from build123d import *

# Parameters (mm, degrees)
SKETCH1_W           = 80
SKETCH1_H           = 80
BOSS_EXTRUDE1_DEPTH = 2.5
SKETCH2_W           = 80
SKETCH2_H           = 80
SKETCH2_W_2         = 75
SKETCH2_H_2         = 75
BOSS_EXTRUDE2_DEPTH = 16
BOSS_EXTRUDE3_REACH = 93.336
SKETCH4_W           = 5
SKETCH4_H           = 2
CUT_EXTRUDE2_DEPTH  = 2.5


with BuildPart() as part:
    # Sketch1 → Boss-Extrude1 (new body)
    with BuildSketch(Plane(origin=(0, 0, 0), x_dir=(1, 0, 0), z_dir=(0, 1, 0))):
        Rectangle(SKETCH1_W, SKETCH1_H)
    extrude(amount=BOSS_EXTRUDE1_DEPTH)

    # Sketch2 → Boss-Extrude2 (add)
    with BuildSketch(Plane(origin=(0, 2.5, 0), x_dir=(1, 0, 0), z_dir=(0, 1, 0))):
        Rectangle(SKETCH2_W, SKETCH2_H)
        Rectangle(SKETCH2_W_2, SKETCH2_H_2, mode=Mode.SUBTRACT)
    extrude(amount=BOSS_EXTRUDE2_DEPTH)

    # Sketch4 → Boss-Extrude3 (add, up to next)
    with BuildSketch(Plane.XY.offset(40), mode=Mode.PRIVATE) as boss_extrude3_sk1:
        with Locations((-37.5, 17.5)):
            Rectangle(SKETCH4_W, SKETCH4_H)
    boss_extrude3_tool1 = extrude(boss_extrude3_sk1.sketch, amount=-BOSS_EXTRUDE3_REACH, mode=Mode.PRIVATE) - part.part
    # Sketch4 → Boss-Extrude3 (add, up to next)
    with BuildSketch(Plane.XY.offset(40), mode=Mode.PRIVATE) as boss_extrude3_sk2:
        with Locations((37.5, 17.5)):
            Rectangle(SKETCH4_W, SKETCH4_H)
    boss_extrude3_tool2 = extrude(boss_extrude3_sk2.sketch, amount=-BOSS_EXTRUDE3_REACH, mode=Mode.PRIVATE) - part.part
    add(boss_extrude3_tool1.solids().sort_by_distance((-37.5, 17.5, 40))[0])
    add(boss_extrude3_tool2.solids().sort_by_distance((37.5, 17.5, 40))[0])

    # Sketch5 → Cut-Extrude2 (cut)
    with BuildSketch(Plane(origin=(0, 0, -40), x_dir=(-1, 0, 0), z_dir=(0, 0, -1))):
        Polygon((-32.2, 18.5), (-35, 18.5), (-35, 16.5), (-37.5, 16.5), (-37.5, 14.2), (-32.2, 14.2), align=None)
        Polygon((35, 18.5), (32.2, 18.5), (32.2, 14.2), (37.5, 14.2), (37.5, 16.5), (35, 16.5), align=None)
    extrude(amount=-CUT_EXTRUDE2_DEPTH, mode=Mode.SUBTRACT)


solid = part.part
Could you check a few things on this model? Use its own coordinates, in mm. A direction names the side the tool comes from. Round coordinates to 2 decimals unless told otherwise and drop trailing zeros. Write each loop counter-clockwise with the first axis right and the second up, starting at its lowest first coordinate (ties: lowest second). Pieces come first, ordered by that corner, then holes. Notation, with made-up numbers: (0, 24.5) - (24, 24.5) arc R32 cw to (24, 59.5) - close; hole circle Ø9 at (-24, -33.75). An arc over 180 degrees is marked (long way). Use a Markdown table: item, result.
Q1. I want a section at B-B (x = 20.5). List the corners of the cut face in (y, z) for me, plus the area to 3 significant figures.
Output values:
| item | result |
|---|---|
| outline | (0, -40) - (18.5, -40) - (18.5, -37.5) - (2.5, -37.5) - (2.5, 37.5) - (18.5, 37.5) - (18.5, 40) - (0, 40) - close |
| area | 280 mm2 |
Q2. Thinking about a two-plate mould opening in Z: for faces 1 (the flat face through (-1, 9, 40)), 2 (the flat face through (40, 9, 1)), 3 (the flat face through (-37.5, 9, -1)), which applies, released by +Z, released by -Z, zero draft, split by the parting line, or undercut?
Output values:
| item | result |
|---|---|
| face 1 | released by +Z |
| face 2 | zero draft |
| face 3 | undercut |
Q3. I want a section at A-A (y = 11.75). List the corners of the cut face in (x, z) for me.
Output values:
| item | result |
|---|---|
| outline | (-40, -40) - (40, -40) - (40, 40) - (-40, 40) - close; hole (-37.5, -37.5) - (37.5, -37.5) - (37.5, 37.5) - (-37.5, 37.5) - close |
Q4. For faces 4 (the flat face through (-35, 14.2, -39)), 5 (the flat face through (-40, 9, 1)), 6 (the flat face through (32.2, 16, -39)), which set-ups out of +Z, -Z, +X, -X, +Y, -Y let a thin tool reach every point of the face, with its end or its side?
Output values:
| item | result |
|---|---|
| face 4 | -Z |
| face 5 | +Z, -Z, -X, +Y, -Y |
| face 6 | -Z, +Y |
Q5. For pin 1 (5 mm diameter, centred on x = 3.5, z = 8.5, fed in from +Y); pin 2 (0.8 mm diameter, centred on x = -34, z = -38.5, fed in from +Y), each with a flat end and sliding along its axis, tell me the tip position at first contact or that it passes through.
Output values:
| item | result |
|---|---|
| pin 1 | y = 2.5 |
| pin 2 | y = 14.2 |
Q6. Please list where these lines run through material, in increasing order: L1, parallel to Z at x = -9.5, y = 9.25; L2, parallel to Y at x = -36, z = 18.
Output values:
| item | result |
|---|---|
| L1 | -40 to -37.5, 37.5 to 40 |
| L2 | 0 to 2.5, 16.5 to 18.5 |
Q7. I want a section at C-C (z = -35). List the corners of the cut face in (x, y) for me, plus the area to 3 significant figures.
Output values:
| item | result |
|---|---|
| outline | (-40, 0) - (40, 0) - (40, 18.5) - (35, 18.5) - (35, 16.5) - (37.5, 16.5) - (37.5, 2.5) - (-37.5, 2.5) - (-37.5, 16.5) - (-35, 16.5) - (-35, 18.5) - (-40, 18.5) - close |
| area | 290 mm2 |
